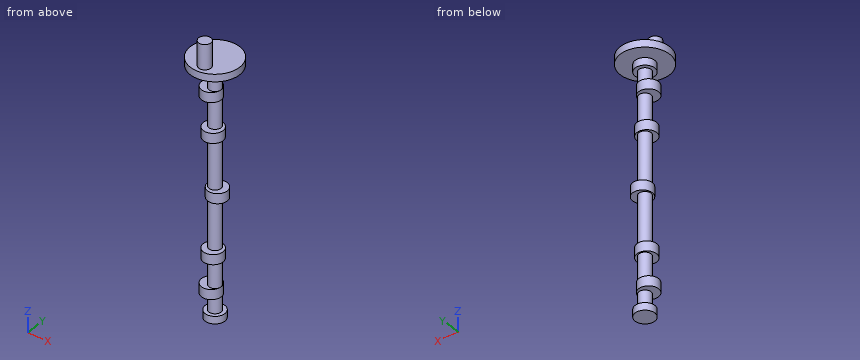
from build123d import *

# Parameters (mm, degrees)
F0_R          = 4
F1_DEPTH      = 3
F1_DEPTH_BACK = 1
F2_R          = 2.5
F3_DEPTH      = 98
F5_R          = 4
F6_DEPTH      = 4
F8_R          = 4
F9_DEPTH      = 4
F11_R         = 4
F12_DEPTH     = 4
F14_R         = 4
F15_DEPTH     = 4
F17_R         = 4
F18_DEPTH     = 4
F20_START     = 2
F19_R         = 10
F20_DEPTH     = 3
F21_R         = 2.5
F22_DEPTH     = 10
F24_R         = 2
F24_R_2       = 1
F25_DEPTH     = 1
F26_R         = 4
F26_R_2       = 2.5
F27_DEPTH     = 3


# Not quite as in the source:
# - a feature names something its author has since deleted; it is built from what else it names


with BuildPart() as f1:
    # F0 (on Top) → F1 (new body, two sides)
    with BuildSketch(Plane.XY) as f1_sk:
        Circle(F0_R)
    extrude(amount=F1_DEPTH)
    extrude(f1_sk.sketch, amount=-F1_DEPTH_BACK)

    # F2 (on Top) → F3 (join)
    with BuildSketch(Plane.XY):
        Circle(F2_R)
    extrude(amount=-F3_DEPTH)

    # F5 (on offset) → F6 (join)
    with BuildSketch(Plane.XY.offset(-50)):
        with Locations((1, 0)):
            Circle(F5_R)
    extrude(amount=F6_DEPTH)

    # F8 (on offset) → F9 (join)
    with BuildSketch(Plane.XY.offset(-26)):
        with Locations((0, -1)):
            Circle(F8_R)
    extrude(amount=F9_DEPTH)

    # F11 (on offset) → F12 (join)
    with BuildSketch(Plane.XY.offset(-11)):
        with Locations((-1.5, 0)):
            Circle(F11_R)
    extrude(amount=F12_DEPTH)

    # F14 (on offset) → F15 (join)
    with BuildSketch(Plane.XY.offset(-74)):
        with Locations((0, -1)):
            Circle(F14_R)
    extrude(amount=F15_DEPTH)

    # F17 (on offset) → F18 (join)
    with BuildSketch(Plane.XY.offset(-89)):
        with Locations((-1.5, 0)):
            Circle(F17_R)
    extrude(amount=F18_DEPTH)

    # F19 (on Top) → F20 (join)
    with BuildSketch(Plane.XY.offset(F20_START)):
        Circle(F19_R)
    extrude(amount=F20_DEPTH)

    # F21 (on face) → F22 (join)
    with BuildSketch(Plane.XY.offset(5)):
        with Locations((0.3544102503, -5.989523635)):
            Circle(F21_R)
    extrude(amount=F22_DEPTH)

    # F24 (on offset) → F25 (cut)
    with BuildSketch(Plane.XY.offset(-1)):
        Circle(F24_R)
        Circle(F24_R_2, mode=Mode.SUBTRACT)
    extrude(amount=-F25_DEPTH, mode=Mode.SUBTRACT)

    # F26 (on face) → F27 (join)
    with BuildSketch(Plane(origin=(0, 0, -98), x_dir=(1, 0, 0), z_dir=(0, 0, -1))):
        Circle(F26_R)
        Circle(F26_R_2, mode=Mode.SUBTRACT)
    extrude(amount=-F27_DEPTH)


solid = f1.part
Could you check a few things on this model? Use its own coordinates, in mm. Coordinates: 2 decimals unless noted, no trailing zeros. Loops run counter-clockwise (first coordinate to the right, second up) from the corner with the lowest first, then second, coordinate; pieces in that order, holes last.
1. Imagine slicing it at B-B (y = -7.5). Please give me the cut outline in (x, z).
2. Imagine slicing it at A-A (z = 1). Please give me the cut outline in (x, y).
3. For P1, Ø4, axis at x = -2, y = 0, coming from the +Z side; P2, Ø8, axis at x = 1, z = -37.5, coming from the -Y side; P3, Ø6, axis at x = -3.5, z = -6.5, coming from the +Y side, each with a flat end and sliding along its axis, tell me the tip position at first contact or that it passes through.
4. I need wall thicknesses on L1, parallel to Y at x = 0, z = -1.75; L2, parallel to Z at x = 1, y = -4.5; L3, parallel to Z at x = -3.5, y = -0.5. Which ranges of each line are inside material? Lowest first, please.
5. Imagine slicing it at C-C (x = -8.5). Please give me the cut outline in (y, z), and give its area (3 significant figures).
6. Imagine slicing it at D-D (z = -28.5). Please give me the cut outline in (x, y).
Computed values:
1. outline: (-6.61, 2) - (6.61, 2) - (6.61, 5) - (2.35, 5) - (2.35, 15) - (-1.64, 15) - (-1.64, 5) - (-6.61, 5) - close
2. outline: circle Ø8 at (0, 0)
3. P1: stops at z = 5
3. P2: stops at y = -2.5
3. P3: stops at y = 4
4. L1: y = -2.5 to -2, -1 to 1, 2 to 2.5
4. L2: z = -74 to -70, -26 to -22, 2 to 15
4. L3: z = -98 to -95, -89 to -85, -74 to -70, -26 to -22, -11 to -7, -1 to 5
5. outline: (-5.27, 2) - (5.27, 2) - (5.27, 5) - (-5.27, 5) - close
5. area: 31.6 mm2
6. outline: circle Ø5 at (0, 0)
